Could you check a few things on this model? Use its own coordinates, in mm. Give positions to 0.01 mm unless a question says otherwise; leave off trailing zeros. Order: outer loops, then holes, each group sorted by start corner. A loop starts at its lowest first (then second) coordinate and runs counter-clockwise, first axis right, second up. Notation, with made-up numbers: (35.5, -36) -> (50.5, -36) arc R20 ccw to (50.5, -14) -> close; hole circle Ø7 at (46.5, 51.25). An arc over 180 degrees is marked (long way). One line per item, written item: value.
Autodesk Inventor part; units mm, degrees
ref_plane "MONTAGEPLATTE_XY" through (0, 0, 0) normal (0, 0, 1) x (1, 0, 0)
ref_plane "MONTAGEPLATTE_YZ" through (0, 0, 0) normal (1, 0, 0) x (0, 1, 0)
ref_plane "MONTAGEPLATTE_ZX" through (0, 0, 0) normal (0, 1, 0) x (0, 0, 1)
sketch "Sketch_7" plane through (0, 0, 0) normal (0, 0, 1) x (1, 0, 0)
  line L0 (-87.5, 117.5) -> (-87.5, -117.5)
  line L1 (-87.5, -117.5) -> (-74.5, -117.5)
  line L2 (-74.5, -117.5) -> (-66, -126)
  line L3 (-66, -126) -> (-50, -126)
  line L4 (-50, -126) -> (-47, -129)
  line L5 (-47, -129) -> (-47, -139.5)
  line L6 (-47, -139.5) -> (-44, -142.5)
  line L7 (-44, -142.5) -> (-28.3, -142.5)
  line L8 (-28.3, -142.5) -> (-28.3, -128)
  arc A0 (-21.7, -128) -> (-28.3, -128) centre (-25, -128) ccw
  line L9 (-21.7, -128) -> (-21.7, -142.5)
  line L10 (-21.7, -142.5) -> (21.7, -142.5)
  line L11 (21.7, -142.5) -> (21.7, -128)
  arc A1 (28.3, -128) -> (21.7, -128) centre (25, -128) ccw
  line L12 (28.3, -128) -> (28.3, -142.5)
  line L13 (28.3, -142.5) -> (44, -142.5)
  line L14 (44, -142.5) -> (47, -139.5)
  line L15 (47, -139.5) -> (47, -129)
  line L16 (47, -129) -> (50, -126)
  line L17 (50, -126) -> (66, -126)
  line L18 (66, -126) -> (74.5, -117.5)
  line L19 (74.5, -117.5) -> (87.5, -117.5)
  line L20 (87.5, -117.5) -> (87.5, 117.5)
  line L21 (87.5, 117.5) -> (74.5, 117.5)
  line L22 (74.5, 117.5) -> (66, 126)
  line L23 (66, 126) -> (50, 126)
  line L24 (50, 126) -> (47, 129)
  line L25 (47, 129) -> (47, 139.5)
  line L26 (47, 139.5) -> (44, 142.5)
  line L27 (44, 142.5) -> (28.3, 142.5)
  line L28 (28.3, 142.5) -> (28.3, 128)
  arc A2 (21.7, 128) -> (28.3, 128) centre (25, 128) ccw
  line L29 (21.7, 128) -> (21.7, 142.5)
  line L30 (21.7, 142.5) -> (-21.7, 142.5)
  line L31 (-21.7, 142.5) -> (-21.7, 128)
  arc A3 (-28.3, 128) -> (-21.7, 128) centre (-25, 128) ccw
  line L32 (-28.3, 128) -> (-28.3, 142.5)
  line L33 (-28.3, 142.5) -> (-44, 142.5)
  line L34 (-44, 142.5) -> (-47, 139.5)
  line L35 (-47, 139.5) -> (-47, 129)
  line L36 (-47, 129) -> (-50, 126)
  line L37 (-50, 126) -> (-66, 126)
  line L38 (-66, 126) -> (-74.5, 117.5)
  line L39 (-74.5, 117.5) -> (-87.5, 117.5)
  circle A4 centre (75, 100) radius 2.6
  circle A5 centre (75, -100) radius 2.6
  circle A6 centre (-75, 100) radius 2.6
  circle A7 centre (-75, -100) radius 2.6
extrude "Extrusion1" add sketch "Sketch_7" along normal blind 2
ref_plane "MONTAGEPLATTE_XY" through (0, 0, 0) normal (0, 0, 1) x (1, 0, 0)
ref_plane "MONTAGEPLATTE_YZ" through (0, 0, 0) normal (1, 0, 0) x (0, 1, 0)
ref_plane "MONTAGEPLATTE_ZX" through (0, 0, 0) normal (0, 1, 0) x (0, 0, 1)
properties part number "1301.000_6_(1)"
1) If I drill on line 1 along Y through (x, z) = (75, 1.5); line 2 along X through (y, z) = (-101.5, 0.75); line 3 along Y through (x, z) = (76, 1.3), over which ranges is the centre line in solid material (lowest first)?
Answer below:
line 1: y = -117.5 to -102.6, -97.4 to 97.4, 102.6 to 117.5
line 2: x = -87.5 to -77.12, -72.88 to 72.88, 77.12 to 87.5
line 3: y = -117.5 to -102.4, -97.6 to 97.6, 102.4 to 117.5
2) Suppose I cut it at B-B, the plane x = 25. Write out the boundary of the cut face in (y, z).
Answer below:
outline: (-124.7, 0) -> (124.7, 0) -> (124.7, 2) -> (-124.7, 2) -> close
3) Suppose I cut it at A-A, the plane z = 1.25. State how many separate pieces and enclosed holes the cut face has, then the cut area to 3 significant figures.
Answer below:
separate pieces: 1
enclosed holes: 4
area: 46,100 mm2
4) For P1, Ø0.6, axis at y = -136.5, z = 1, coming from the +X side; P2, Ø1, axis at x = 57.5, z = 1, coming from the -Y side; P3, Ø0.6, axis at y = 137.5, z = 1, coming from the -X side, each with a flat end and sliding along its axis, tell me the tip position at first contact or that it passes through.
Answer below:
P1: stops at x = 47
P2: stops at y = -126
P3: stops at x = -47
5) We'd pull the mould along Y, two halves only. Please class faces 1 (the flat face through (-70, 122, 1)), 2 (the cylindrical face through (73.084, 98.243, 0.986)), 3 (the flat face through (70, -122, 1)): +Y half, -Y half, draft (parallel to the pull), parting line (faces both ways), or undercut.
Answer below:
face 1: +Y half
face 2: undercut
face 3: -Y half
